For this review, take the finished solid that the model builds, in its own axes (mm). A direction names the side the tool comes from. Coordinates: 2 decimals unless noted, no trailing zeros. Order: outer loops, then holes, each group sorted by start corner. A loop starts at its lowest first (then second) coordinate and runs counter-clockwise, first axis right, second up.
from build123d import *

# Parameters (mm, degrees)
BOSS_EXTRUDE1_DEPTH            = 40.5
BOSS_EXTRUDE2_DEPTH            = 11.5
CUT_EXTRUDE1_DEPTH             = 38.5
CUT_EXTRUDE2_DEPTH             = 38.5
CUT_EXTRUDE3_DEPTH             = 38.5
CUT_EXTRUDE4_DEPTH             = 38.5
CUT_EXTRUDE5_DEPTH             = 38.5
CUT_EXTRUDE6_DEPTH             = 38.5
CUT_EXTRUDE7_DEPTH             = 50
F_18_0_18_DIAMETER_HOLE1_D     = 18
F_18_0_18_DIAMETER_HOLE1_DEPTH = 52
F_2_45_2_45_DIAMETER_HOLE1_D   = 2.45
F_4_0_4_DIAMETER_HOLE1_D       = 4
F_4_0_4_DIAMETER_HOLE1_DEPTH   = 3
F_4_0_4_DIAMETER_HOLE2_D       = 4
F_4_0_4_DIAMETER_HOLE2_DEPTH   = 3
F_4_0_4_DIAMETER_HOLE3_D       = 4
F_4_0_4_DIAMETER_HOLE3_DEPTH   = 3


with BuildPart() as part:
    # Sketch1 → Boss-Extrude1 (new body)
    with BuildSketch(Plane.XZ.offset(0.5)):
        Polygon((64.951905284, 37.5), (-64.951905284, 37.5), (0, -75), align=None)
    extrude(amount=-BOSS_EXTRUDE1_DEPTH)

    # Sketch4 → Boss-Extrude2 (add)
    with BuildSketch(Plane(origin=(0, 40, 0), x_dir=(-1, 0, 0), z_dir=(0, 1, 0))):
        Polygon((0, -61), (-52.827549631, 30.5), (52.827549631, 30.5), align=None)
    extrude(amount=BOSS_EXTRUDE2_DEPTH)

    # Sketch2 → Cut-Extrude1 (cut)
    with BuildSketch(Plane(origin=(0, 40, 0), x_dir=(-1, 0, 0), z_dir=(0, 1, 0))):
        Polygon((-0.899647383, -59.441765024), (-51.827549631, 28.767949192), (-49.94764189, 17.511853471), (-9.707758354, -52.185669302), align=None)
    extrude(amount=-CUT_EXTRUDE1_DEPTH, mode=Mode.SUBTRACT)

    # Sketch3 → Cut-Extrude2 (cut)
    with BuildSketch(Plane(origin=(0, 40, 0), x_dir=(-1, 0, 0), z_dir=(0, 1, 0))):
        Polygon((-50.827549631, 30.5), (51.028254843, 30.5), (40.340234991, 34.5), (-40.139530918, 34.5), align=None)
    extrude(amount=-CUT_EXTRUDE2_DEPTH, mode=Mode.SUBTRACT)

    # Sketch5 → Cut-Extrude3 (cut)
    with BuildSketch(Plane(origin=(0, 40, 0), x_dir=(-1, 0, 0), z_dir=(0, 1, 0))):
        Polygon((50.047994507, 17.685669302), (51.827549631, 28.767949192), (1, -59.267949192), (9.707758354, -52.185669302), align=None)
    extrude(amount=-CUT_EXTRUDE3_DEPTH, mode=Mode.SUBTRACT)

    # Sketch6 → Cut-Extrude4 (cut)
    with BuildSketch(Plane(origin=(0, 40, 0), x_dir=(-1, 0, 0), z_dir=(0, 1, 0))):
        Polygon((-42.340236152, 35), (-60.621778265, 35), (-51.481007209, 19.16772011), (-52.827549631, 30.5), align=None)
    extrude(amount=-CUT_EXTRUDE4_DEPTH, mode=Mode.SUBTRACT)

    # Sketch7 → Cut-Extrude5 (cut)
    with BuildSketch(Plane(origin=(0, 40, 0), x_dir=(-1, 0, 0), z_dir=(0, 1, 0))):
        Polygon((60.621778265, 35), (51.481007209, 19.16772011), (52.827549631, 30.5), (42.340234991, 35), align=None)
    extrude(amount=-CUT_EXTRUDE5_DEPTH, mode=Mode.SUBTRACT)

    # Sketch8 → Cut-Extrude6 (cut)
    with BuildSketch(Plane(origin=(0, 40, 0), x_dir=(-1, 0, 0), z_dir=(0, 1, 0))):
        Polygon((0, -70), (-9.140771056, -54.16772011), (0, -61), (9.140771056, -54.16772011), align=None)
    extrude(amount=-CUT_EXTRUDE6_DEPTH, mode=Mode.SUBTRACT)

    # Sketch9 → Cut-Extrude7 (cut)
    with BuildSketch(Plane(origin=(0, 51.5, 0), x_dir=(-1, 0, 0), z_dir=(0, 1, 0))):
        Polygon((47.631397208, 27.5), (-47.631397208, 27.5), (0, -55), align=None)
    extrude(amount=-CUT_EXTRUDE7_DEPTH, mode=Mode.SUBTRACT)

    # Ø18.0 (18) Diameter Hole1
    with Locations(Plane(origin=(0, -0.5, 0), x_dir=(-1, 0, 0), z_dir=(0, -1, 0))):
        with Locations((0, 0)):
            Hole(F_18_0_18_DIAMETER_HOLE1_D / 2, depth=F_18_0_18_DIAMETER_HOLE1_DEPTH)

    # Ø2.45 (2.45) Diameter Hole1 (through all)
    with Locations(Plane(origin=(0, 1.5, 0), x_dir=(1, 0, 0), z_dir=(0, 1, 0))):
        with Locations((13.95, 13.95), (-13.95, -13.95), (13.95, -13.95), (-13.95, 13.95)):
            Hole(F_2_45_2_45_DIAMETER_HOLE1_D / 2)

    # Ø4.0 (4) Diameter Hole1
    with Locations(Plane.XY.offset(37.5)):
        with Locations((59.951905284, 35), (-59.951905284, 35)):
            Hole(F_4_0_4_DIAMETER_HOLE1_D / 2, depth=F_4_0_4_DIAMETER_HOLE1_DEPTH)

    # Ø4.0 (4) Diameter Hole2
    with Locations(Plane(origin=(-32.475952642, 0, -18.75), x_dir=(-0.5000000000000003, 0, 0.8660254037844385), z_dir=(-0.8660254037844385, 0, -0.5000000000000003))):
        with Locations((-59.951905284, 35), (59.951905284, 35)):
            Hole(F_4_0_4_DIAMETER_HOLE2_D / 2, depth=F_4_0_4_DIAMETER_HOLE2_DEPTH)

    # Ø4.0 (4) Diameter Hole3
    with Locations(Plane(origin=(32.475952642, 0, -18.75), x_dir=(-0.499999999999999, 0, -0.8660254037844394), z_dir=(0.8660254037844394, 0, -0.499999999999999))):
        with Locations((59.951905284, 35), (-59.951905284, 35)):
            Hole(F_4_0_4_DIAMETER_HOLE3_D / 2, depth=F_4_0_4_DIAMETER_HOLE3_DEPTH)


solid = part.part
1. The part is to be moulded in two halves that separate along Z. For faces 1 (the face through (1, 1.5, 33)), 2 (the face through (-32.93, 19.47, -17.96)), 3 (the face through (-15, -0.5, -5)), say which applies: +Z half, -Z half, draft (parallel to the pull), parting line (faces both ways), or undercut.
Answer below:
face 1: undercut
face 2: -Z half
face 3: draft
2. Take a section at B-B, the plane z = 0. Give the boundary of the cut face in (x, y), plus the area to 3 significant figures.
Answer below:
outline: (-43.3, -0.5) - (-9, -0.5) - (-9, 1.5) - (-31.75, 1.5) - (-31.75, 51.5) - (-35.22, 51.5) - (-35.22, 1.5) - (-39.84, 1.5) - (-39.84, 40) - (-43.3, 40) - close; (9, -0.5) - (43.3, -0.5) - (43.3, 40) - (39.84, 40) - (39.84, 1.5) - (35.22, 1.5) - (35.22, 51.5) - (31.75, 51.5) - (31.75, 1.5) - (9, 1.5) - close
area: 750 mm2
3. Take a section at D-D, the plane y = 43.5. Give the boundary of the cut face in (x, z).
Answer below:
outline: (-52.83, 30.5) - (0, -61) - (52.83, 30.5) - close; hole (-47.63, 27.5) - (0, -55) - (47.63, 27.5) - close
4. Machinability: for faces 4 (the face through (-2.401, 35.088, -68.306)), 5 (the face through (26.044, 26.15, -15.89)), which of the approach directions +Z, -Z, +X, -X, +Y, -Y give a long, thin tool a straight path to every point of the face, cutting with its end or side? Answer none if there is none.
Answer below:
face 4: none
face 5: +Y
5. To check wall thickness, follow L1, parallel to X at y = 37, z = 26; L2, parallel to Z at x = -13.95, y = 0.95 (3 decimals); L3, parallel to X at y = 37.5, z = -4.5. State the ranges of each line that lie inside material, in increasing order.
Answer below:
L1: x = -58.31 to -55.43, -52.29 to -51.38, -50.23 to -46.77, 46.77 to 50.23, 51.37 to 52.29, 55.43 to 58.31
L2: z = -50.838 to -15.175, -12.725 to 12.725, 15.175 to 37.5
L3: x = -40.7 to -37.24, -32.62 to -29.16, 29.16 to 32.62, 37.24 to 40.7
6. Take a section at C-C, the plane x = 20. Give the boundary of the cut face in (y, z), plus the area to 3 significant figures.
Answer below:
outline: (-0.5, -40.36) - (40, -40.36) - (40, -34.36) - (1.5, -34.36) - (1.5, -26.36) - (51.5, -26.36) - (51.5, -20.36) - (1.5, -20.36) - (1.5, 27.5) - (51.5, 27.5) - (51.5, 30.5) - (1.5, 30.5) - (1.5, 34.5) - (40, 34.5) - (40, 37.5) - (-0.5, 37.5) - close
area: 952 mm2
7. Take a section at A-A, the plane y = 25. Give the number of separate pieces and of enclosed holes in the cut face, plus the area to 3 significant figures.
Answer below:
separate pieces: 1
enclosed holes: 7
area: 2,040 mm2
8. Clearance check with flat-ended pins moving along their axes: pin 1 Ø14.5 at (x, y) = (50.5, 23) entering from -Z; pin 2 Ø14.5 at (x, z) = (0, 0) entering from -Y; pin 3 Ø2.5 at (x, y) = (-59.95, 35) entering from -Z; pin 4 Ø12.5 at (x, z) = (-3.5, -65) entering from +Y. State where each tip first meets the part, or that it passes through.
Answer below:
pin 1: stops at z = -0.09
pin 2: passes through
pin 3: stops at z = 26.67
pin 4: stops at y = 51.5
